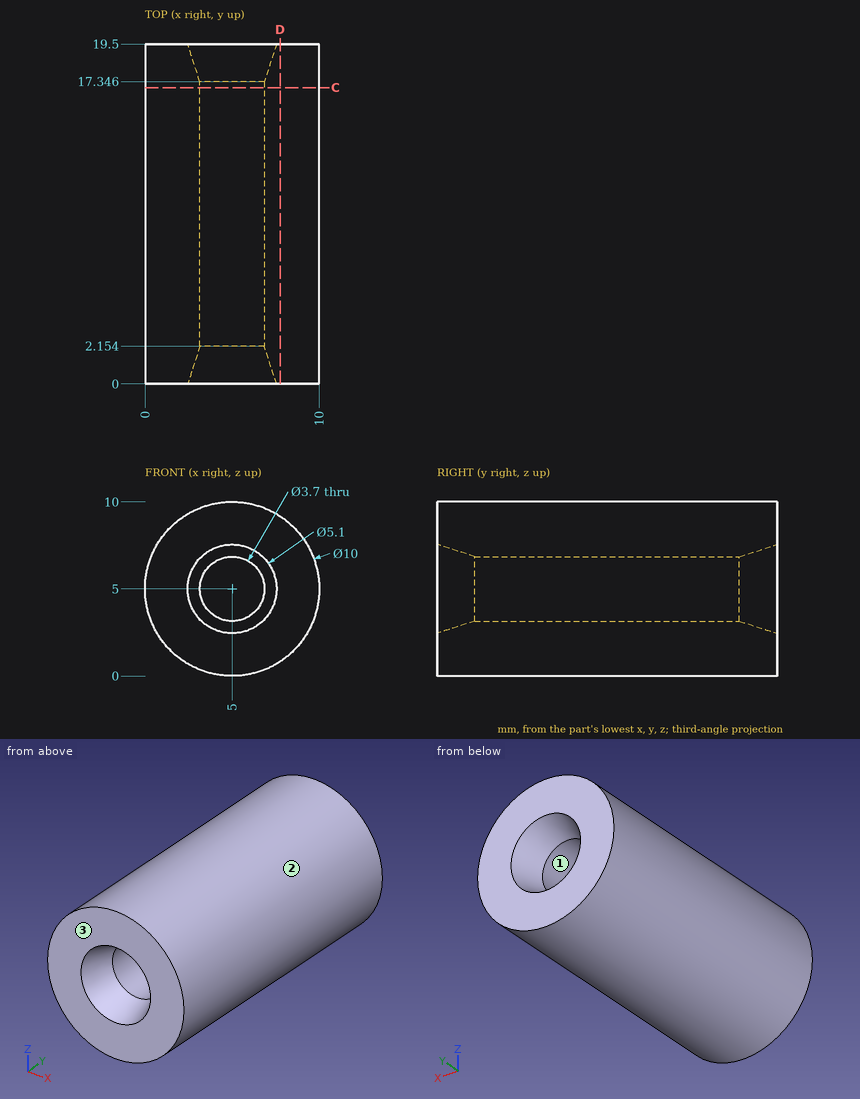
The figure shows three views and two pictorial views of one solid part (mm, origin at its lowest corner). Answer the questions. Give positions to 0.01 mm unless a question says otherwise; leave off trailing zeros. Order: outer loops, then holes, each group sorted by start corner. A loop starts at its lowest first (then second) coordinate and runs counter-clockwise, first axis right, second up. Notation, with made-up numbers: (-35, 83.5) -> (10, 83.5) arc R23 cw to (10, 114.5) -> close; hole circle Ø7 at (36.25, -14). An arc over 180 degrees is marked (long way). Answer as a JSON object with one key per item and string values. Group by question number.
Item 1: Determine the mould class of the marked faces 1, 2 and 3 for opening direction Z: pulls with the +Z half, pulls with the -Z half, needs draft (parallel to the pull), parting line crosses it, or undercut.
Item 2: The part is cut by section C-C on y = 17. Write down the section's boundary in (x, z).
Item 3: Consider L1, parallel to X at y = 7, z = 5; L2, parallel to X at y = 13.75, z = 3.5 (1 decimal). Determine where each line is inside the solid, lowest interval first. Write a range as from..to.
Item 4: The part is cut by section D-D on x = 7.75. Write down the section's boundary in (y, z).
Item 5: Flat-ended cylindrical pins translate along their axes: pin 1 (6 mm diameter, centred on y = 5.5, z = 8.5, fed in from -X) (1 decimal); pin 2 (3 mm diameter, centred on x = 7, y = 5.5, fed in from +Z) (1 decimal); pin 3 (1.5 mm diameter, centred on y = 15, z = 8, fed in from -X) (1 decimal). Find the tip coordinate at first contact, or state that the pin passes through.
Result set:
{
 "1": {"face 1": "undercut", "face 2": "parting line crosses it", "face 3": "needs draft"},
 "2": {"outline": "circle Ø10 at (5, 5); hole circle Ø3.7 at (5, 5)"},
 "3": {"L1": "0..3.15, 6.85..10", "L2": "0.2..3.9, 6.1..9.8"},
 "4": {"outline": "(0, 0.82) -> (19.5, 0.82) -> (19.5, 9.18) -> (0, 9.18) -> close"},
 "5": {"pin 1": "x = 0", "pin 2": "z = 10", "pin 3": "x = 0.5"}
}
